The model under review builds one solid part; all positions refer to its coordinate system, in mm. A direction names the side the tool comes from. Coordinates: 2 decimals unless noted, no trailing zeros. Loops run counter-clockwise (first coordinate to the right, second up) from the corner with the lowest first, then second, coordinate; pieces in that order, holes last. Notation, with made-up numbers: M 65,86.25 L 109,86.25 A20 ccw 109,99.25 Z; hole C 48,89.5 d11. An arc over 180 degrees is marked long. Use one line per item in the form item = value.
Autodesk Inventor part; units mm, degrees
ref_plane "YZ Plane" through (0, 0, 0) normal (1, 0, 0) x (0, 1, 0)
ref_plane "XZ Plane" through (0, 0, 0) normal (0, 1, 0) x (-1, 0, 0)
ref_plane "XY Plane" through (0, 0, 0) normal (0, 0, 1) x (1, 0, 0)
sketch "Sketch1" plane through (0, 0, 0) normal (0, 0, 1) x (1, 0, 0)
  circle A0 centre (0, 0) radius 63.5
  dimension "d0" = 127
extrude "Extrusion1" add sketch "Sketch1" along normal blind 25.4
sketch "Sketch2" plane through (0, 0, 25.4) normal (0, 0, 1) x (1, 0, 0)
  circle A0 centre (0, 0) radius 28.575
  dimension "d3" = 57.15
extrude "Extrusion2" add sketch "Sketch2" along normal blind 19.05
sketch "Sketch3" plane through (0, 0, 44.45) normal (0, 0, 1) x (1, 0, 0)
  circle A0 centre (0, 0) radius 15.875
  dimension "d6" = 31.75
extrude "Extrusion3" cut sketch "Sketch3" against normal through all
sketch "Sketch4" plane through (0, 0, 25.4) normal (0, 0, 1) x (1, 0, 0)
  line L0 (0, 0) -> (0, 38.1)
  line L1 (0, 38.1) -> (0, -38.1)
  line L2 (0, -38.1) -> (6.35, -38.1)
  line L3 (6.35, -38.1) -> (6.35, -63.1817)
  circle A0 centre (0, 0) radius 63.5
  line L4 (0, -38.1) -> (-6.35, -38.1)
  line L5 (-6.35, -38.1) -> (-6.35, -80.9216)
  line L6 (-6.35, -80.9216) -> (6.35, -63.1817)
  line L7 (0, 38.1) -> (6.35, 38.1)
  line L8 (6.35, 38.1) -> (6.35, 68.5855)
  line L9 (0, 38.1) -> (-6.35, 38.1)
  line L10 (-6.35, 38.1) -> (-6.35, 68.5855)
  line L11 (-6.35, 68.5855) -> (6.35, 68.5855)
  dimension "d9" = 38.1
  dimension "d10" = 76.2
  dimension "d11" = 6.35
  dimension "d12" = 6.35
  dimension "d13" = 6.35
  dimension "d14" = 6.35
extrude "Extrusion4" cut sketch "Sketch4" against normal through all contours L9 L10 A0 L8 L7 | L2 L3 A0 L5 L4 | A0 L10 L11 L8 | L6 L5 A0
sketch "Sketch5" plane through (0, 0, 25.4) normal (0, 0, 1) x (1, 0, 0)
  line L0 (0, 0) -> (38.1, 0)
  line L1 (38.1, 0) -> (-38.1, 0)
  line L2 (-38.1, 0) -> (-38.1, 6.35)
  line L3 (-38.1, 6.35) -> (-99.0804, 6.35)
  line L4 (-38.1, 0) -> (-38.1, -6.35)
  line L5 (-38.1, -6.35) -> (-95.4724, -6.35)
  line L6 (-95.4724, -6.35) -> (-99.0804, 6.35)
  line L7 (38.1, 0) -> (38.1, -6.35)
  line L8 (38.1, -6.35) -> (92.4195, -6.35)
  line L9 (38.1, 0) -> (38.1, 6.35)
  line L10 (38.1, 6.35) -> (95.1949, 6.35)
  line L11 (95.1949, 6.35) -> (92.4195, -6.35)
  dimension "d17" = 38.1
  dimension "d18" = 76.2
  dimension "d19" = 6.35
  dimension "d20" = 6.35
  dimension "d21" = 6.35
  dimension "d22" = 6.35
extrude "Extrusion5" cut sketch "Sketch5" against normal through all
sketch "Sketch6" plane through (0, 0, 25.4) normal (0, 0, 1) x (1, 0, 0)
  point P0 (0, 0)
sketch "Sketch7" plane through (0, 0, 25.4) normal (0, 0, 1) x (1, 0, 0)
  line L0 (0, 0) -> (31.75, 0)
  line L1 (0, 0) -> (0, 31.75)
  line L2 (0, 31.75) -> (124.8927, 31.75)
  line L3 (0, 0) -> (0, -31.75)
  line L4 (0, 0) -> (-31.75, 0)
  line L5 (-31.75, 0) -> (-145.867, 0)
  line L6 (0, 31.75) -> (-126.7995, 31.75)
  line L7 (0, -31.75) -> (-134.9032, -31.75)
  line L8 (0, -31.75) -> (128.2295, -31.75)
  line L9 (-31.75, -31.75) -> (-31.75, -121.3175)
  line L10 (-31.75, -121.3175) -> (-134.9032, -31.75)
  line L11 (28.575, -31.75) -> (28.575, -121.3175)
  line L12 (28.575, -121.3175) -> (128.2295, -31.75)
  line L13 (28.575, 31.75) -> (28.575, 107.95)
  line L14 (28.575, 107.95) -> (124.8927, 31.75)
  line L15 (-126.7995, 31.75) -> (-31.75, 99.6281)
  line L16 (-31.75, 99.6281) -> (-31.75, 31.75)
  dimension "d25" = 31.75
  dimension "d26" = 31.75
  dimension "d27" = 31.75
  dimension "d28" = 31.75
  dimension "d29" = 76.2
extrude "Extrusion6" cut sketch "Sketch7" against normal through all
properties part number "3-3" material "Iron, Malleable"
1. Add section A-A (y = -46.5). State the section outline as (x, z) points (3 decimals), then the cut area to 3 significant figures.
Response values:
outline = M -31.75,0 L -6.35,0 L -6.35,25.4 L -31.75,25.4 Z; M 6.35,0 L 28.575,0 L 28.575,25.4 L 6.35,25.4 Z
area = 1,210 mm^2
2. Add section D-D (x = 0). State the section outline as (y, z) points (3 decimals).
Response values:
outline = M -38.1,0 L -15.875,0 L -15.875,44.45 L -28.575,44.45 L -28.575,25.4 L -38.1,25.4 Z; M 15.875,0 L 38.1,0 L 38.1,25.4 L 28.575,25.4 L 28.575,44.45 L 15.875,44.45 Z
3. Add section B-B (x = -44.5). State the section outline as (y, z) points, then the cut area to 3 significant figures.
Response values:
outline = M -31.75,0 L -6.35,0 L -6.35,25.4 L -31.75,25.4 Z; M 6.35,0 L 31.75,0 L 31.75,25.4 L 6.35,25.4 Z
area = 1,290 mm^2
4. Insertion check: P1, Ø20.5, axis at x = 43, z = 13, coming from the -Y side; P2, Ø12.5, axis at y = -52, z = 15, coming from the -X side; P3, Ø12, axis at x = 18, z = 17.5, coming from the +Y side. Each pin has a flat end and moves straight along its axis. Give the tip position at first contact, or say it passes through.
Response values:
P1 = -31.75
P2 = -31.75
P3 = 62.36
5. Wall thickness on line 1 along Y through (x, z) = (0, 35) (3 decimals); line 2 along X through (y, z) = (45, 11) (3 decimals); line 3 along Y through (x, z) = (0, 22) (3 decimals): over which ranges is each line inside the solid? List them lowest first. Write a range as from..to.
Response values:
line_1 = -28.575..-15.875, 15.875..28.575
line_2 = -31.75..-6.35, 6.35..28.575
line_3 = -38.1..-15.875, 15.875..38.1
6. Machinability: for faces 1 (the face through (42, 31.75, 13)), 2 (the face through (-6.35, -50, 13)), 3 (the face through (0, 38.1, 13)), 4 (the face through (-43, -31.75, 13)), which of the approach directions +Z, -Z, +X, -X, +Y, -Y give a long, thin tool a straight path to every point of the face, cutting with its end or side? Answer none if there is none.
Response values:
face_1 = +Z, -Z, +X, +Y
face_2 = +Z, -Z, -Y
face_3 = +Z, -Z, +Y
face_4 = +Z, -Z, -X, -Y
